from build123d import *

# Parameters (mm, degrees)
BOSS_EXTRUDE1_DEPTH      = 27.1
BOSS_EXTRUDE1_DEPTH_BACK = 9.9
SKETCH2_W                = 20
SKETCH2_H                = 40.6
SKETCH1_R                = 2.83646338
SKETCH1_R_2              = 2.25
BOSS_EXTRUDE2_DEPTH      = 2
FILLET1_R                = 3
SKETCH3_R                = 3
BOSS_EXTRUDE3_DEPTH      = 5


with BuildPart() as part:
    # Sketch2 → Boss-Extrude1 (new, two sides: drawn at the far end of the back side and taken through both)
    with BuildSketch(Plane.XY.offset(-BOSS_EXTRUDE1_DEPTH_BACK)):
        Rectangle(SKETCH2_W, SKETCH2_H)
    extrude(amount=BOSS_EXTRUDE1_DEPTH + BOSS_EXTRUDE1_DEPTH_BACK)

    # Sketch1 → Boss-Extrude2 (add)
    with BuildSketch(Plane.XY):
        with BuildLine():
            Line((-5, -27.7), (5, -27.7))
            ThreePointArc((5, -27.7), (8.535533906, -26.235533906), (10, -22.7))
            Line((10, -22.7), (10, 22.7))
            ThreePointArc((10, 22.7), (8.535533906, 26.235533906), (5, 27.7))
            Line((5, 27.7), (-5, 27.7))
            ThreePointArc((-5, 27.7), (-8.535533906, 26.235533906), (-10, 22.7))
            Line((-10, 22.7), (-10, -22.7))
            ThreePointArc((-10, -22.7), (-8.535533906, -26.235533906), (-5, -27.7))
        make_face()
        with Locations((0, 9.8)):
            Circle(SKETCH1_R, mode=Mode.SUBTRACT)
        with Locations((-5, 24.3)):
            Circle(SKETCH1_R_2, mode=Mode.SUBTRACT)
        with Locations(Location((5, 24.3, 0), (0, 0, 180))):
            Circle(SKETCH1_R_2, mode=Mode.SUBTRACT)
        with Locations((5, -24.3)):
            Circle(SKETCH1_R_2, mode=Mode.SUBTRACT)
        with Locations(Location((-5, -24.3, 0), (0, 0, 180))):
            Circle(SKETCH1_R_2, mode=Mode.SUBTRACT)
    extrude(amount=BOSS_EXTRUDE2_DEPTH)

    # Fillet1
    fillet1_edges = [part.edges().sort_by_distance(p)[0] for p in [
        (10, 0, -9.9),
        (0, 20.3, -9.9),
        (-10, 0, -9.9),
        (0, -20.3, -9.9),
    ]]
    fillet(fillet1_edges, radius=FILLET1_R)

    # Sketch3 → Boss-Extrude3 (add)
    with BuildSketch(Plane(origin=(0, 0, -9.9), x_dir=(-1, 0, 0), z_dir=(0, 0, -1))):
        with Locations(Location((0, 9.8, 0), (0, 0, 180))):
            Circle(SKETCH3_R)
    extrude(amount=BOSS_EXTRUDE3_DEPTH)


solid = part.part
Could you check a few things on this model? Use its own coordinates, in mm. A direction names the side the tool comes from. Coordinates: 2 decimals unless noted, no trailing zeros. Order: outer loops, then holes, each group sorted by start corner. A loop starts at its lowest first (then second) coordinate and runs counter-clockwise, first axis right, second up. Notation, with made-up numbers: (-5, 52.25) -> (34, 52.25) arc R26 cw to (34, 91.25) -> close; hole circle Ø10 at (-36, 8). An arc over 180 degrees is marked (long way). One line per item, written item: value. Start each with the question number.
1) Imagine slicing it at C-C on y = 15.5. List the corners of the cut face in (x, z) for me.
2) If I drill on L1, parallel to Y at x = -5, z = 0.6; L2, parallel to X at y = 24, z = 1; L3, parallel to Y at x = 7.5, z = 9, over which ranges is the centre line in solid material (lowest first)? Write a range as [from, to].
3) Which directions (+Z, -Z, +X, -X, +Y, -Y) give clear straight access to the entire face, cutting with the end or side of a thin tool? Please do faces 4 (the flat face through (0, 20.3, 14)), 5 (the flat face through (0, 20.3, -3)), 6 (the cylindrical face through (-8.57, -26.2, 0.99)), 7 (the flat face through (0, -24, 2)), 8 (the flat face through (0, -20.3, -3)).
4) We'd pull the mould along X, two halves only. Please class faces 1 (the cylindrical face through (8.57, 26.2, 0.99)), 2 (the flat face through (0, -24, 0)), 3 (the cylindrical face through (-6.038, -22.304, 0.986)): +X half, -X half, draft (parallel to the pull), parting line (faces both ways), or undercut.
5) Imagine slicing it at B-B on y = 24.3. List the corners of the cut face in (x, z) for me, plus the area to 3 significant figures.
6) I'm going to push flat-ended pins straight in: pin 1 (1 mm diameter, centred on x = 5, z = -5.5, fed in from -Y); pin 2 (2 mm diameter, centred on x = -3.5, z = -3.5, fed in from +Y); pin 3 (4 mm diameter, centred on x = -5, y = 24.3, fed in from +Z); pin 4 (7 mm diameter, centred on x = 2, y = -8, fed in from -Z). Where does each tip first touch, or does it pass through?
7) Imagine slicing it at D-D on x = 0. List the corners of the cut face in (y, z) for me.
8) Imagine slicing it at A-A on x = 4. List the corners of the cut face in (y, z) for me.
Answer list:
1. outline: (-10, -6.9) arc R3 ccw to (-7, -9.9) -> (7, -9.9) arc R3 ccw to (10, -6.9) -> (10, 27.1) -> (-10, 27.1) -> close
2. L1: y = [-27.7, -26.55], [-22.05, 22.05], [26.55, 27.7]
2. L2: x = [-9.83, -7.23], [-2.77, 2.77], [7.23, 9.83]
2. L3: y = [-20.3, 20.3]
3. face 4: +Z, +X, -X, +Y
3. face 5: -Z, +X, -X, +Y
3. face 6: +Z, -Z, -X, -Y
3. face 7: +Z, +X, -X, -Y
3. face 8: -Z, +X, -X, -Y
4. face 1: +X half
4. face 2: draft
4. face 3: undercut
5. outline: (-9.74, 0) -> (-7.25, 0) -> (-7.25, 2) -> (-9.74, 2) -> close; (-2.75, 0) -> (2.75, 0) -> (2.75, 2) -> (-2.75, 2) -> close; (7.25, 0) -> (9.74, 0) -> (9.74, 2) -> (7.25, 2) -> close
5. area: 20.9 mm2
6. pin 1: stops at y = -20.3
6. pin 2: stops at y = 20.3
6. pin 3: passes through
6. pin 4: stops at z = -9.9
7. outline: (-27.7, 0) -> (-20.3, 0) -> (-20.3, -6.9) arc R3 ccw to (-17.3, -9.9) -> (6.8, -9.9) -> (6.8, -14.9) -> (12.8, -14.9) -> (12.8, -9.9) -> (17.3, -9.9) arc R3 ccw to (20.3, -6.9) -> (20.3, 0) -> (27.7, 0) -> (27.7, 2) -> (20.3, 2) -> (20.3, 27.1) -> (-20.3, 27.1) -> (-20.3, 2) -> (-27.7, 2) -> close
8. outline: (-27.7, 0) -> (-26.32, 0) -> (-26.32, 2) -> (-27.7, 2) -> close; (-22.28, 0) -> (-20.3, 0) -> (-20.3, -6.9) arc R3 ccw to (-17.3, -9.9) -> (17.3, -9.9) arc R3 ccw to (20.3, -6.9) -> (20.3, 0) -> (22.28, 0) -> (22.28, 2) -> (20.3, 2) -> (20.3, 27.1) -> (-20.3, 27.1) -> (-20.3, 2) -> (-22.28, 2) -> close; (26.32, 0) -> (27.7, 0) -> (27.7, 2) -> (26.32, 2) -> close
